For this review, take the finished solid that the model builds, in its own axes (mm). A direction names the side the tool comes from. Round coordinates to 2 decimals unless told otherwise and drop trailing zeros. Order: outer loops, then holes, each group sorted by start corner. A loop starts at its lowest first (then second) coordinate and runs counter-clockwise, first axis right, second up. Notation, with made-up numbers: (-36, 23.5) - (-22, 23.5) arc R18 ccw to (-22, 52.5) - close; hole circle Ø2 at (2.25, -13.75). An arc over 180 degrees is marked (long way). One line per item, written item: value.
```python
from build123d import *

# Parameters (mm, degrees)
CROQUIS1_R              = 3.1
SALIENTE_EXTRUIR1_DEPTH = 6
CROQUIS2_W              = 6.826394781
CROQUIS2_H              = 2.350070334
CORTAR_EXTRUIR1_DEPTH   = 7
REDONDEO1_R             = 1
REDONDEO2_R             = 0.5


with BuildPart() as part:
    # Croquis1 → Saliente-Extruir1 (new body)
    with BuildSketch(Plane(origin=(0, 0, 0), x_dir=(1, 0, 0), z_dir=(0, 1, 0))):
        with BuildLine():
            Line((-10.05, 7.45), (-7.01, 7.45))
            Line((-7.01, 7.45), (-7.01, 1.614093831))
            Line((-7.01, 1.614093831), (-3.71, 1.614093831))
            Line((-3.71, 1.614093831), (-3.71, 7.45))
            Line((-3.71, 7.45), (10.05, 7.45))
            ThreePointArc((10.05, 7.45), (16.5, 0), (10.05, -7.45))
            Line((10.05, -7.45), (-3.5, -7.45))
            Line((-3.5, -7.45), (-3.5, -1.614093831))
            Line((-3.5, -1.614093831), (-7.3, -1.614093831))
            Line((-7.3, -1.614093831), (-7.3, -7.45))
            Line((-7.3, -7.45), (-10.05, -7.45))
            ThreePointArc((-10.05, -7.45), (-17.5, 0), (-10.05, 7.45))
        make_face()
        with Locations((8.97248062, 0)):
            Circle(CROQUIS1_R, mode=Mode.SUBTRACT)
    extrude(amount=SALIENTE_EXTRUIR1_DEPTH)

    # Croquis2 → Cortar-Extruir1 (cut)
    with BuildSketch(Plane(origin=(0, 6, 0), x_dir=(1, 0, 0), z_dir=(0, 1, 0))):
        with Locations((-11.209462468, 0.149210815)):
            Rectangle(CROQUIS2_W, CROQUIS2_H)
    extrude(amount=-CORTAR_EXTRUIR1_DEPTH, mode=Mode.SUBTRACT)

    # Redondeo1
    redondeo1_edges = [part.edges().sort_by_distance(p)[0] for p in [
        (-7.01, 3, -1.614093831),
        (-3.71, 3, -1.614093831),
        (-3.5, 3, 1.614093831),
        (-7.3, 3, 1.614093831),
    ]]
    fillet(redondeo1_edges, radius=REDONDEO1_R)

    # Redondeo2
    redondeo2_edges = [part.edges().sort_by_distance(p)[0] for p in [
        (-7.796265078, 3, -1.324245982),
        (-7.796265078, 3, 1.025824352),
        (-14.622659859, 3, 1.025824352),
        (-14.622659859, 3, -1.324245982),
    ]]
    fillet(redondeo2_edges, radius=REDONDEO2_R)


solid = part.part
```
Item 1: For P1, Ø1, axis at x = 11, y = 4.5, coming from the +Z side; P2, Ø2, axis at x = -5, y = 4.5, coming from the +Z side; P3, Ø5, axis at x = 8.97, z = 0, coming from the -Y side; P4, Ø2.5, axis at y = 3.5, z = -4.5, coming from the -X side, all flat-tipped, find the tip position at first contact; note any pin that passes through.
Returned:
P1: z = 7.37
P2: z = 1.75
P3: through
P4: x = -16.75
Item 2: Machinability: for faces 5 (the cylindrical face through (-7, 3, 1.9)), 6 (the flat face through (-7.01, 3, -5)), 7 (the flat face through (-11, 3, 1.026)), which of the approach directions +Z, -Z, +X, -X, +Y, -Y give a long, thin tool a straight path to every point of the face, cutting with its end or side? Answer none if there is none.
Returned:
face 5: +Z, +Y, -Y
face 6: -Z, +Y, -Y
face 7: +Y, -Y
Item 3: Take a section at D-D (z = 4.75). Write out the cut boundary in (x, y), plus the area to 3 significant figures.
Returned:
outline: (-15.79, 0) - (-7.3, 0) - (-7.3, 6) - (-15.79, 6) - close; (-3.5, 0) - (14.81, 0) - (14.81, 6) - (-3.5, 6) - close
area: 161 mm^2
Item 4: Take a section at B-B (y = 2.95). Write out the cut boundary in (x, z).
Returned:
outline: (-10.05, -7.45) - (-7.01, -7.45) - (-7.01, -2.61) arc R1 cw to (-6.01, -1.61) - (-4.71, -1.61) arc R1 cw to (-3.71, -2.61) - (-3.71, -7.45) - (10.05, -7.45) arc R7.53 ccw to (10.05, 7.45) - (-3.5, 7.45) - (-3.5, 2.61) arc R1 cw to (-4.5, 1.61) - (-6.3, 1.61) arc R1 cw to (-7.3, 2.61) - (-7.3, 7.45) - (-10.05, 7.45) arc R7.45 ccw to start; hole (-14.62, -0.82) arc R0.5 ccw to (-14.12, -1.32) - (-8.3, -1.32) arc R0.5 ccw to (-7.8, -0.82) - (-7.8, 0.53) arc R0.5 ccw to (-8.3, 1.03) - (-14.12, 1.03) arc R0.5 ccw to (-14.62, 0.53) - close; hole circle Ø6.2 at (8.97, 0)
Item 5: Take a section at A-A (z = 0). Write out the cut boundary in (x, y), plus the area to 3 significant figures.
Returned:
outline: (-17.5, 0) - (-14.62, 0) - (-14.62, 6) - (-17.5, 6) - close; (-7.8, 0) - (5.87, 0) - (5.87, 6) - (-7.8, 6) - close; (12.07, 0) - (16.5, 0) - (16.5, 6) - (12.07, 6) - close
area: 126 mm^2
Item 6: Take a section at C-C (x = 6.5). Write out the cut boundary in (y, z), plus the area to 3 significant figures.
Returned:
outline: (0, -7.45) - (6, -7.45) - (6, -1.87) - (0, -1.87) - close; (0, 1.87) - (6, 1.87) - (6, 7.45) - (0, 7.45) - close
area: 67.0 mm^2
Item 7: The part is to be moulded in two halves that separate along Z. For faces 1 (the flat face through (-3.5, 3, 5)), 2 (the flat face through (-9, 3, -7.45)), 3 (the flat face through (-14.623, 3, 0)), 4 (the flat face through (-11, 3, -1.324)), say which applies: +Z half, -Z half, draft (parallel to the pull), parting line (faces both ways), or undercut.
Returned:
face 1: draft
face 2: -Z half
face 3: undercut
face 4: undercut
Item 8: Wall thickness on line 1 (X direction, y = 4.6, z = 0); line 2 (X direction, y = 5.15, z = -2.5); line 3 (Z direction, x = -9, y = 3.2): over which ranges is each line inside the solid? List them lowest first.
Returned:
line 1: -17.5 to -14.62, -7.8 to 5.87, 12.07 to 16.5
line 2: -17.07 to -7, -3.72 to 7.14, 10.81 to 16.07
line 3: -7.45 to -1.32, 1.03 to 7.45
